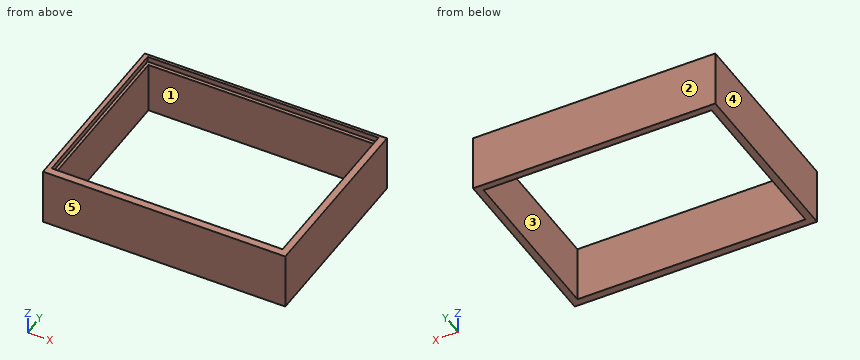
from build123d import *

# Parameters (mm, degrees)
F0_W     = 215.9
F0_H     = 165.1
F1_DEPTH = 50.8
F2_W     = 203.2
F2_H     = 152.4
F3_DEPTH = 50.8
F4_W     = 152.4
F4_H     = 4.8418088436
F5_DEPTH = 2.54
F6_W     = 205.74
F6_H     = 4.8418088436
F7_DEPTH = 3.302


with BuildPart() as f1:
    # F0 (on Top) → F1 (new body)
    with BuildSketch(Plane.XY):
        with Locations((107.95, 82.55)):
            Rectangle(F0_W, F0_H)
    extrude(amount=F1_DEPTH)

    # F2 (on face) → F3 (cut)
    with BuildSketch(Plane(origin=(0, 0, 0), x_dir=(1, 0, 0), z_dir=(0, 0, -1))):
        with Locations((108.1436636686, -83.0071964197)):
            Rectangle(F2_W, F2_H)
    extrude(amount=-F3_DEPTH, mode=Mode.SUBTRACT)

    # F4 (on face) → F5 (cut)
    with BuildSketch(Plane.YZ.offset(6.5436636686)):
        with Locations((83.0071964197, 48.3790955782)):
            Rectangle(F4_W, F4_H)
    extrude(amount=-F5_DEPTH, mode=Mode.SUBTRACT)

    # F6 (on face) → F7 (cut)
    with BuildSketch(Plane.XZ.offset(-159.2071964197)):
        with Locations((106.8736636686, 48.3790955782)):
            Rectangle(F6_W, F6_H)
    extrude(amount=-F7_DEPTH, mode=Mode.SUBTRACT)


solid = f1.part
The listing builds one solid part. Answer for the finished solid, in the listing's coordinates (mm). Face numbers are marked on the shaded views. A direction names the side the tool comes from. Round coordinates to 2 decimals unless told otherwise and drop trailing zeros. Write each loop counter-clockwise with the first axis right and the second up, starting at its lowest first coordinate (ties: lowest second). Pieces come first, ordered by that corner, then holes. Notation, with made-up numbers: (-2, 12) - (37, 12) arc R25 cw to (37, 40) - close; hole circle Ø10 at (30, -6.5). An arc over 180 degrees is marked (long way). Use a Markdown table: item, result. Add a question column.
1. A tool of negligible diameter and unlimited length cuts with its end or side. For the marked faces 1 and 2, from which of +Z, -Z, +X, -X, +Y, -Y can it reach the whole face along a straight path? Write none if from no direction.
2. For a pull along Y with two mould halves and no side action, classify the marked faces 3, 4 and 5 as +Y half, -Y half, draft (parallel to the pull), parting line (faces both ways), or undercut.
3. The part is cut by section B-B (y = 31.5). Write down the section's boundary in (x, z).
4. The part is cut by section C-C (z = 15.5). Write down the section's boundary in (x, y).
5. The part is cut by section A-A (x = 185.5). Write down the section's boundary in (y, z), and give its area (3 significant figures).
6. Consider line 1 (X direction, y = 95.5, z = 5.5); line 2 (Y direction, x = 27.5, z = 16.5); line 3 (X direction, y = 103, z = 46). Determine where each line is inside the solid, lowest interval first.
Reported:
| question | item | result |
|---|---|---|
| 1 | face 1 | +Z, -Z |
| 1 | face 2 | +Z, -Z, +X, -X, +Y |
| 2 | face 3 | undercut |
| 2 | face 4 | draft |
| 2 | face 5 | -Y half |
| 3 | outline | (0, 0) - (6.54, 0) - (6.54, 45.96) - (4, 45.96) - (4, 50.8) - (0, 50.8) - close; (209.74, 0) - (215.9, 0) - (215.9, 50.8) - (209.74, 50.8) - close |
| 4 | outline | (0, 0) - (215.9, 0) - (215.9, 165.1) - (0, 165.1) - close; hole (6.54, 6.81) - (209.74, 6.81) - (209.74, 159.21) - (6.54, 159.21) - close |
| 5 | outline | (0, 0) - (6.81, 0) - (6.81, 50.8) - (0, 50.8) - close; (159.21, 0) - (165.1, 0) - (165.1, 50.8) - (162.51, 50.8) - (162.51, 45.96) - (159.21, 45.96) - close |
| 5 | area | 629 mm^2 |
| 6 | line 1 | 0 to 6.54, 209.74 to 215.9 |
| 6 | line 2 | 0 to 6.81, 159.21 to 165.1 |
| 6 | line 3 | 0 to 4, 209.74 to 215.9 |
